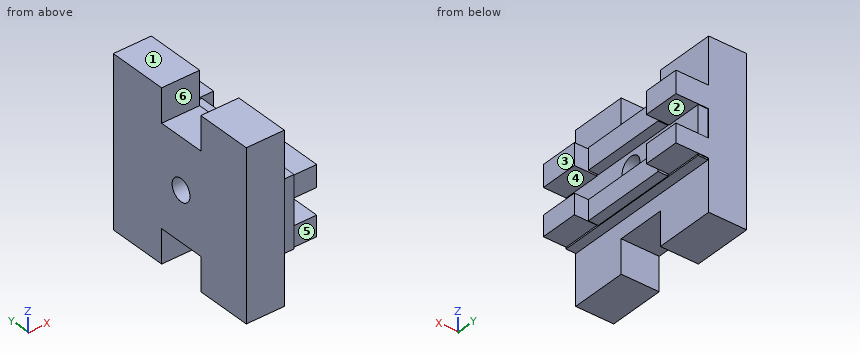
```python
from build123d import *

# Parameters (mm, degrees)
F1_DEPTH = 25.4
F2_W     = 109.303277
F2_H     = 47.219016
F3_DEPTH = 32.004
F4_W     = 25.649838
F4_H     = 14.573772
F4_H_2   = 13.699345
F4_W_2   = 0.291478
F4_H_3   = 14.865246
F4_W_3   = 24.192456
F4_W_4   = 24.483934
F4_H_4   = 12.533444
F5_DEPTH = 47.244
F6_W     = 57.712132
F6_H     = 14.282296
F6_H_2   = 13.407867
F7_DEPTH = 38.608
F8_R     = 7.375251
F9_DEPTH = 65.278


with BuildPart() as f1:
    # F0 (on Right) → F1 (new body)
    with BuildSketch(Plane.YZ):
        Polygon((-16.322624, 56.109019), (-53.922951, 56.109019), (-53.922951, -55.526067), (-16.322624, -55.526067), (-16.322624, -33.082449), (16.031148, -33.082449), (16.031148, -55.526067), (55.963278, -55.526067), (55.963278, 56.109019), (16.031148, 56.109019), (16.031148, 33.665407), (-16.322624, 33.665407), align=None)
    extrude(amount=F1_DEPTH)

    # F2 (on Right) → F3 (join)
    with BuildSketch(Plane.YZ):
        with Locations((0.874429, 1.457378)):
            Rectangle(F2_W, F2_H)
    extrude(amount=F3_DEPTH)

    # F4 (on Right) → F5 (join)
    with BuildSketch(Plane.YZ):
        with Locations((-40.806558, 17.342787)):
            Rectangle(F4_W, F4_H)
        with Locations((-40.806558, -14.282296)):
            Rectangle(F4_W, F4_H_2)
        with Locations((55.817539, 17.488524)):
            Rectangle(F4_W_2, F4_H_3)
        with Locations((43.575572, 17.488524)):
            Rectangle(F4_W_3, F4_H_3)
        with Locations((43.721311, -14.865246)):
            Rectangle(F4_W_4, F4_H_4)
    extrude(amount=F5_DEPTH)

    # F6 (on Right) → F7 (join)
    with BuildSketch(Plane.YZ):
        with Locations((1.748853, 17.488525)):
            Rectangle(F6_W, F6_H)
        with Locations((1.748853, -15.010982)):
            Rectangle(F6_W, F6_H_2)
    extrude(amount=F7_DEPTH)

    # F8 (on Right) → F9 (cut)
    with BuildSketch(Plane.YZ):
        Circle(F8_R)
    extrude(amount=F9_DEPTH, mode=Mode.SUBTRACT)


solid = f1.part
```
CAD build for the part. Positions are in the model's coordinates, mm. Face numbers are marked on the shaded views. A direction names the side the tool comes from. Give positions to 0.01 mm unless a question says otherwise; leave off trailing zeros. Order: outer loops, then holes, each group sorted by start corner. A loop starts at its lowest first (then second) coordinate and runs counter-clockwise, first axis right, second up. Notation, with made-up numbers: M -1,-5 L 24,-5 A37 ccw 24,33 Z; hole C 31,28 d8. An arc over 180 degrees is marked long. Put each result on its own line as item: value. Start each with the question number.
(1) Which spindle directions (+Z, -Z, +X, -X, +Y, -Y) get a long thin tool onto all of the face, cutting with end or side? Do the marked faces 4, 5 and 6. Say none if no direction does.
(2) Saw through at C-C, the plane x = 7. Write the cut outline in (y, z), then the cut area to 3 significant figures.
(3) Mould opens along Z. For the marked faces 1, 2 and 3 say: +Z half, -Z half, draft (parallel to the pull), parting line (faces both ways), or undercut.
(4) Flat gauge pins, fed straight in: pin 1 Ø2 at (x, y) = (35.5, 3) entering from +Z; pin 2 Ø10 at (y, z) = (33, -37.5) entering from +X; pin 3 Ø17 at (x, y) = (42.5, -43.5) entering from -Z. Where does each tip first touch, or does it go through?
(5) Saw through at B-B, the plane y = 0. Write the cut outline in (x, z), then the cut area to 3 significant figures.
(6) Saw through at A-A, the plane z = 46. Write the cut outline in (x, y).
(7) Drill centre lines: line 1 along Z through (x, y) = (22, 0); line 2 along Y through (x, z) = (19, 0); line 3 along Y through (x, z) = (8, 39). Where is each one in solid material? Low to high.
(8) Saw through at D-D, the plane y = 44. Write the cut outline in (x, z).
Check result:
1. face 4: +X, +Y, -Y
1. face 5: +Z, -Z, +X, -Y
1. face 6: +Z, +X, -X
2. outline: M -53.92,-55.53 L -16.32,-55.53 L -16.32,-33.08 L 16.03,-33.08 L 16.03,-55.53 L 55.96,-55.53 L 55.96,56.11 L 16.03,56.11 L 16.03,33.67 L -16.32,33.67 L -16.32,56.11 L -53.92,56.11 Z; hole C 0,0 d14.75
2. area: 10,600 mm2
3. face 1: +Z half
3. face 2: undercut
3. face 3: draft
4. pin 1: stops at z = 24.63
4. pin 2: stops at x = 25.4
4. pin 3: stops at z = -21.13
5. outline: M 0,-33.08 L 25.4,-33.08 L 25.4,-22.15 L 32,-22.15 L 32,-21.71 L 38.61,-21.71 L 38.61,-8.31 L 32,-8.31 L 32,-7.38 L 0,-7.38 Z; M 0,7.38 L 32,7.38 L 32,10.35 L 38.61,10.35 L 38.61,24.63 L 32,24.63 L 32,25.07 L 25.4,25.07 L 25.4,33.67 L 0,33.67 Z
5. area: 1,720 mm2
6. outline: M 0,-53.92 L 25.4,-53.92 L 25.4,-16.32 L 0,-16.32 Z; M 0,16.03 L 25.4,16.03 L 25.4,55.96 L 0,55.96 Z
7. line 1: z = -33.08 to -7.38, 7.38 to 33.67
7. line 2: y = -53.92 to -7.38, 7.38 to 55.96
7. line 3: y = -53.92 to -16.32, 16.03 to 55.96
8. outline: M 0,-55.53 L 25.4,-55.53 L 25.4,-22.15 L 32,-22.15 L 32,-21.13 L 47.24,-21.13 L 47.24,-8.6 L 32,-8.6 L 32,10.06 L 47.24,10.06 L 47.24,24.92 L 32,24.92 L 32,25.07 L 25.4,25.07 L 25.4,56.11 L 0,56.11 Z
